For this review, take the finished solid that the model builds, in its own axes (mm). Face numbers are marked on the shaded views. Give positions to 0.01 mm unless a question says otherwise; leave off trailing zeros. Write each loop counter-clockwise with the first axis right and the second up, starting at its lowest first coordinate (ties: lowest second). Pieces come first, ordered by that corner, then holes. Notation, with made-up numbers: M -25.75,88 L -2.75,88 A21 cw -2.75,108 Z; hole C 75,-38 d5. An arc over 180 degrees is marked long. One line per item, written item: value. Start each with the question number.
Item 1: To check wall thickness, follow probe 1 along X at (y, z) = (19, 11); probe 2 along Z at (x, y) = (-13.5, 17.5); probe 3 along Y at (x, z) = (8, 37.5). State the ranges of each line that lie inside material, in increasing order.
Item 2: Consider section C-C, the plane x = -31.5. Write out the cut boundary in (y, z), and give its area (3 significant figures).
Item 3: Consider section A-A, the plane y = 26. Give the number of separate pieces and of enclosed holes in the cut face, and give its area (3 significant figures).
Item 4: Consider section D-D, the plane z = -35.5. Write out the cut boundary in (x, y).
Item 5: Clearance check with flat-ended pins moving along their axes: pin 1 Ø7 at (x, z) = (-80, 0.1) entering from +Y; pin 2 Ø14 at (y, z) = (15.5, -9.5) entering from +X; pin 3 Ø1.5 at (x, y) = (-10.5, 11) entering from -Z. State where each tip first meets the part, or that it passes through.
Item 6: Mouldability with a two-part tool opening along X and no side actions: class the marked faces 1, 2, 3 and 4 as released by +X, released by -X, zero draft, split by the parting line, or undercut.
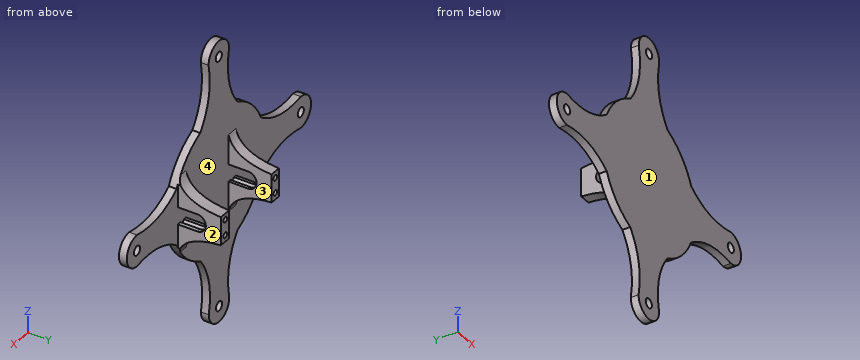
```python
from build123d import *

# Parameters (mm, degrees)
SKIZZE1_R                            = 45
AUFSATZ_LINEAR_AUSTRAGEN1_DEPTH      = 5
SKIZZE3_W                            = 8
SKIZZE3_H                            = 18
AUFSATZ_LINEAR_AUSTRAGEN2_DEPTH      = 27.5
SCHNITT_LINEAR_AUSTRAGEN1_DEPTH      = 70.55
AUFSATZ_LINEAR_AUSTRAGEN3_DEPTH      = 56.7
SCHNITT_LINEAR_AUSTRAGEN2_DEPTH      = 10
SCHNITT_LINEAR_AUSTRAGEN3_DEPTH      = 78.313941464
SCHNITT_LINEAR_AUSTRAGEN3_DEPTH_BACK = 78.313941464
SKIZZE7_W                            = 40.7
SKIZZE7_H                            = 27.5
SCHNITT_LINEAR_START                 = -27.5
SKIZZE8_R                            = 1.75
SCHNITT_LINEAR_AUSTRAGEN4_DEPTH      = 27.5
AUFSATZ_LINEAR_AUSTRAGEN4_DEPTH      = 5
SCHNITT_LINEAR_AUSTRAGEN5_REACH      = 133.363
SKIZZE10_W                           = 0.902438157
SKIZZE10_H                           = 49.081982533
SKIZZE11_R                           = 3
SCHNITT_LINEAR_AUSTRAGEN6_DEPTH      = 14.11


with BuildPart() as part:
    # Skizze1 → Aufsatz-Linear austragen1 (new body)
    with BuildSketch(Plane(origin=(0, 0, 0), x_dir=(1, 0, 0), z_dir=(0, 1, 0))):
        with Locations(Location((0, 0, 0), (0, 0, 270))):
            Circle(SKIZZE1_R)
    extrude(amount=AUFSATZ_LINEAR_AUSTRAGEN1_DEPTH)

    # Skizze3 → Aufsatz-Linear austragen2 (add)
    with BuildSketch(Plane(origin=(0, 5, 0), x_dir=(1, 0, 0), z_dir=(0, 1, 0))):
        with Locations((-12.534256165, -0.183687062)):
            Rectangle(SKIZZE3_W, SKIZZE3_H)
        with Locations((36.165743835, -0.183687062)):
            Rectangle(SKIZZE3_W, SKIZZE3_H)
    extrude(amount=AUFSATZ_LINEAR_AUSTRAGEN2_DEPTH)

    # Skizze4 → Schnitt-Linear austragen1 (cut)
    with BuildSketch(Plane.ZY.offset(16.534256165)):
        with BuildLine():
            Line((-5.316312938, 5), (5.686817911, 5))
            Line((5.686817911, 5), (5.686817911, 17.409920336))
            ThreePointArc((5.686817911, 17.409920336), (0.185252486, 22.91148576), (-5.316312938, 17.409920336))
            Line((-5.316312938, 17.409920336), (-5.316312938, 5))
        make_face()
    extrude(amount=-SCHNITT_LINEAR_AUSTRAGEN1_DEPTH, mode=Mode.SUBTRACT)

    # Skizze5 → Aufsatz-Linear austragen3 (add)
    with BuildSketch(Plane.ZY.offset(16.534256165)):
        with BuildLine():
            Line((-8.816312938, 32.5), (-8.816312938, 5))
            Line((-8.816312938, 5), (-24.357304204, 5))
            add(Edge.make_bspline(
                [(-8.816312938, 32.5), (-10.372494309, 8.167321108), (-24.357304204, 5)],
                knots=[0, 0, 0, 1, 1, 1], degree=2))
        make_face()
        with BuildLine():
            Line((9.183687062, 32.5), (9.183687062, 5))
            Line((9.183687062, 5), (24.724678329, 5))
            add(Edge.make_bspline(
                [(9.183687062, 32.5), (10.739868433, 8.167321108), (24.724678329, 5)],
                knots=[0, 0, 0, 1, 1, 1], degree=2))
        make_face()
    extrude(amount=-AUFSATZ_LINEAR_AUSTRAGEN3_DEPTH)

    # Skizze6 → Schnitt-Linear austragen2 (cut)
    with BuildSketch(Plane.XZ):
        with BuildLine():
            Line((36.037718441, 26.949635426), (42.778201445, 28.630726097))
            Line((42.778201445, 28.630726097), (51.77679317, -24.277660434))
            Line((51.77679317, -24.277660434), (37.77898382, -29.776799822))
            Line((37.77898382, -29.776799822), (35.341876768, -27.855910441))
            ThreePointArc((35.341876768, -27.855910441), (44.996373382, -0.571298967), (36.037718441, 26.949635426))
        make_face()
    extrude(amount=-SCHNITT_LINEAR_AUSTRAGEN2_DEPTH, mode=Mode.SUBTRACT)

    # Skizze7 → Schnitt-Linear austragen3 (cut, two sides: drawn at the far end of the back side and taken through both)
    with BuildSketch(Plane.XY.offset(-8.816312938).offset(-SCHNITT_LINEAR_AUSTRAGEN3_DEPTH_BACK)):
        with Locations((11.815743835, 18.75)):
            Rectangle(SKIZZE7_W, SKIZZE7_H)
    extrude(amount=SCHNITT_LINEAR_AUSTRAGEN3_DEPTH + SCHNITT_LINEAR_AUSTRAGEN3_DEPTH_BACK, mode=Mode.SUBTRACT)

    # Skizze8 → Schnitt-Linear austragen4 (cut)
    with BuildSketch(Plane(origin=(0, 32.5, 0), x_dir=(1, 0, 0), z_dir=(0, 1, 0)).offset(SCHNITT_LINEAR_START)):
        with Locations(Location((-12.984256165, 4.666312938, 0), (0, 0, 270))):
            Circle(SKIZZE8_R)
        with Locations(Location((-12.984256165, -5.033687062, 0), (0, 0, 270))):
            Circle(SKIZZE8_R)
        with Locations(Location((35.81519379, -5.265385311, 0), (0, 0, 270))):
            Circle(SKIZZE8_R)
        with Locations(Location((35.862672939, 4.734501975, 0), (0, 0, 270))):
            Circle(SKIZZE8_R)
    extrude(amount=SCHNITT_LINEAR_AUSTRAGEN4_DEPTH, mode=Mode.SUBTRACT)

    # Skizze9 → Aufsatz-Linear austragen4 (add, through all)
    with BuildSketch(Plane(origin=(0, 5, 0), x_dir=(1, 0, 0), z_dir=(0, 1, 0))):
        with BuildLine():
            Line((-18.254939841, 41.130975814), (18.045289753, 41.130975814))
            add(Edge.make_bspline(
                [(9.895174956, 79.999931323), (5.449457034, 58.022999533), (18.045289753, 41.130975814)],
                knots=[0, 0, 0, 1, 1, 1], degree=2))
            ThreePointArc((9.895174956, 79.999931323), (-0.104825044, 89.999931323), (-10.104825044, 79.999931323))
            add(Edge.make_bspline(
                [(-10.104825044, 79.999931323), (-5.659107122, 58.022999533), (-18.254939841, 41.130975814)],
                knots=[0, 0, 0, 1, 1, 1], degree=2))
        make_face()
        with BuildLine():
            Line((41.130975814, 18.254939841), (41.130975814, -18.045289753))
            add(Edge.make_bspline(
                [(79.999931323, -9.895174956), (58.022999533, -5.449457034), (41.130975814, -18.045289753)],
                knots=[0, 0, 0, 1, 1, 1], degree=2))
            ThreePointArc((79.999931323, -9.895174956), (89.999931323, 0.104825044), (79.999931323, 10.104825044))
            add(Edge.make_bspline(
                [(79.999931323, 10.104825044), (58.022999533, 5.659107122), (41.130975814, 18.254939841)],
                knots=[0, 0, 0, 1, 1, 1], degree=2))
        make_face()
        with BuildLine():
            Line((-18.045289753, -41.130975814), (18.254939841, -41.130975814))
            add(Edge.make_bspline(
                [(10.104825044, -79.999931323), (5.659107122, -58.022999533), (18.254939841, -41.130975814)],
                knots=[0, 0, 0, 1, 1, 1], degree=2))
            ThreePointArc((10.104825044, -79.999931323), (0.104825044, -89.999931323), (-9.895174956, -79.999931323))
            add(Edge.make_bspline(
                [(-9.895174956, -79.999931323), (-5.449457034, -58.022999533), (-18.045289753, -41.130975814)],
                knots=[0, 0, 0, 1, 1, 1], degree=2))
        make_face()
        with BuildLine():
            Line((-41.130975814, 18.045289753), (-41.130975814, -18.254939841))
            add(Edge.make_bspline(
                [(-79.999931323, -10.104825044), (-58.022999533, -5.659107122), (-41.130975814, -18.254939841)],
                knots=[0, 0, 0, 1, 1, 1], degree=2))
            ThreePointArc((-79.999931323, -10.104825044), (-89.999931323, -0.104825044), (-79.999931323, 9.895174956))
            add(Edge.make_bspline(
                [(-79.999931323, 9.895174956), (-58.022999533, 5.449457034), (-41.130975814, 18.045289753)],
                knots=[0, 0, 0, 1, 1, 1], degree=2))
        make_face()
    extrude(amount=-AUFSATZ_LINEAR_AUSTRAGEN4_DEPTH)

    # Schnitt-Linear austragen5: up to this face of the body (flat: up to its plane)
    schnitt_linear_austragen5_end = Plane(part.part.faces().sort_by_distance((-0.703165137, 5, -0.008888692))[0])
    # Skizze10 → Schnitt-Linear austragen5 (cut, up to the picked face)
    with BuildSketch(Plane(origin=(0, 32.5, 0), x_dir=(1, 0, 0), z_dir=(0, 1, 0)), mode=Mode.PRIVATE) as schnitt_linear_austragen5_sk1:
        with Locations((-8.985475244, -0.183687063)):
            Rectangle(SKIZZE10_W, SKIZZE10_H)
    schnitt_linear_austragen5_tool1 = split(extrude(schnitt_linear_austragen5_sk1.sketch, amount=-SCHNITT_LINEAR_AUSTRAGEN5_REACH, mode=Mode.PRIVATE), bisect_by=schnitt_linear_austragen5_end, keep=Keep.BOTH, mode=Mode.PRIVATE)
    add(schnitt_linear_austragen5_tool1.solids().sort_by(Axis((-8.985475, 32.5, 0.183687), (0, -1, 0)))[0], mode=Mode.SUBTRACT)

    # Skizze11 → Schnitt-Linear austragen6 (cut)
    with BuildSketch(Plane(origin=(0, 5, 0), x_dir=(1, 0, 0), z_dir=(0, 1, 0))):
        with Locations(Location((-79.999931323, -0.104825044, 0), (0, 0, 270))):
            Circle(SKIZZE11_R)
        with Locations(Location((-0.104825044, 79.999931323, 0), (0, 0, 270))):
            Circle(SKIZZE11_R)
        with Locations(Location((79.999931323, 0.104825044, 0), (0, 0, 270))):
            Circle(SKIZZE11_R)
        with Locations(Location((0.104825044, -79.999931323, 0), (0, 0, 270))):
            Circle(SKIZZE11_R)
    extrude(amount=-SCHNITT_LINEAR_AUSTRAGEN6_DEPTH, mode=Mode.SUBTRACT)


solid = part.part
```
Model answer:
1. probe 1: x = -16.53 to -9.44, 32.17 to 40.17
1. probe 2: z = -11.63 to -6.34, 6.71 to 12
1. probe 3: y = 0 to 5
2. outline: M 0,-32.14 L 5,-32.14 L 5,32.14 L 0,32.14 Z
2. area: 321 mm2
3. separate pieces: 2
3. enclosed holes: 4
3. area: 254 mm2
4. outline: M -27.65,0 L 27.65,0 L 27.65,5 L -27.65,5 Z
5. pin 1: stops at y = 5
5. pin 2: stops at x = 40.17
5. pin 3: stops at z = -15.7
6. face 1: zero draft
6. face 2: released by +X
6. face 3: undercut
6. face 4: undercut
